```python
from build123d import *

# Parameters (mm, degrees)
BOSS_EXTRUDE1_DEPTH = 5.15
SKETCH2_W           = 4.95
SKETCH2_H           = 2.8
CUT_EXTRUDE1_DEPTH  = 6.15


with BuildPart() as part:
    # Sketch1 → Boss-Extrude1 (new body)
    with BuildSketch(Plane.XY):
        Polygon((-18.1, 1.9), (-18.1, -0.1), (0, -0.1), (18.1, -0.1), (18.1, 1.9), (23.25, 1.9), (23.25, 6.1), (18.1, 6.1), (18.1, 8.1), (-18.1, 8.1), (-18.1, 6.1), (-23.25, 6.1), (-23.25, 1.9), align=None)
    extrude(amount=BOSS_EXTRUDE1_DEPTH)

    # Sketch2 → Cut-Extrude1 (cut, through all)
    with BuildSketch(Plane.XY.offset(5.15)):
        with Locations((-10.575, 4)):
            Rectangle(SKETCH2_W, SKETCH2_H)
        with Locations((10.575, 4)):
            Rectangle(SKETCH2_W, SKETCH2_H)
    extrude(amount=-CUT_EXTRUDE1_DEPTH, mode=Mode.SUBTRACT)


solid = part.part
```
Build history of the part. All positions in model axes, mm. A direction names the side the tool comes from. Give positions to 0.01 mm unless a question says otherwise; leave off trailing zeros. Order: outer loops, then holes, each group sorted by start corner. A loop starts at its lowest first (then second) coordinate and runs counter-clockwise, first axis right, second up. Notation, with made-up numbers: M -10.75,70.25 L 2.25,70.25 A11 ccw 2.25,90.25 Z; hole C 75.5,48.25 d2. An arc over 180 degrees is marked long. Write item = value, one per line. Start each with the question number.
(1) Two-plate mould, pull along Y, no slides. Class faces 1 (the flat face through (21, 6.1, 3)), 2 (the flat face through (-11, 2.6, 3)), 3 (the flat face through (0, 4, 0)): released by +Y, released by -Y, zero draft, split by the parting line, or undercut.
(2) Slice it at D-D on y = 7. Write the cut outline in (x, z).
(3) Probe L1, parallel to X at y = 4, z = 2.3; L2, parallel to Y at x = 10, z = 0.4; L3, parallel to X at y = 6.25, z = 4.95. List the from-to ranges inside material, lowest first. Write a range as [from, to].
(4) Slice it at C-C on z = 0.9. Write the cut outline in (x, y), plus the area to 3 significant figures.
(5) Pin check, flat tips, straight feed: pin 1 Ø0.6 at (y, z) = (1, 3.5) entering from +X; pin 2 Ø1.5 at (x, z) = (-20, 4) entering from +Y. Stop position of each tip, or through.
(6) Slice it at B-B on y = 3.5. Write the cut outline in (x, z).
(7) Slice it at A-A on x = -12.5. Write the cut outline in (y, z).
(8) Which spindle directions (+Z, -Z, +X, -X, +Y, -Y) get a long thin tool onto all of the face, cutting with end or side? Do faces 4 (the flat face through (11, 2.6, 3)), 5 (the flat face through (-21, 6.1, 3)), 6 (the flat face through (21, 1.9, 3)), 7 (the flat face through (-18.1, 1, 3)), 8 (the flat face through (18.1, 7, 3)). Say none if no direction does.
Responses:
q1.face_1 = released by +Y
q1.face_2 = undercut
q1.face_3 = zero draft
q2.outline = M -18.1,0 L 18.1,0 L 18.1,5.15 L -18.1,5.15 Z
q3.L1 = [-23.25, -13.05], [-8.1, 8.1], [13.05, 23.25]
q3.L2 = [-0.1, 2.6], [5.4, 8.1]
q3.L3 = [-18.1, 18.1]
q4.outline = M -23.25,1.9 L -18.1,1.9 L -18.1,-0.1 L 18.1,-0.1 L 18.1,1.9 L 23.25,1.9 L 23.25,6.1 L 18.1,6.1 L 18.1,8.1 L -18.1,8.1 L -18.1,6.1 L -23.25,6.1 Z; hole M -13.05,2.6 L -8.1,2.6 L -8.1,5.4 L -13.05,5.4 Z; hole M 8.1,2.6 L 13.05,2.6 L 13.05,5.4 L 8.1,5.4 Z
q4.area = 312 mm2
q5.pin_1 = 18.1
q5.pin_2 = 6.1
q6.outline = M -23.25,0 L -13.05,0 L -13.05,5.15 L -23.25,5.15 Z; M -8.1,0 L 8.1,0 L 8.1,5.15 L -8.1,5.15 Z; M 13.05,0 L 23.25,0 L 23.25,5.15 L 13.05,5.15 Z
q7.outline = M -0.1,0 L 2.6,0 L 2.6,5.15 L -0.1,5.15 Z; M 5.4,0 L 8.1,0 L 8.1,5.15 L 5.4,5.15 Z
q8.face_4 = +Z, -Z
q8.face_5 = +Z, -Z, -X, +Y
q8.face_6 = +Z, -Z, +X, -Y
q8.face_7 = +Z, -Z, -X, -Y
q8.face_8 = +Z, -Z, +X, +Y
